Here's how the part is built. I have some questions about the finished solid (model axes, mm). Face numbers are marked on the shaded views. A direction names the side the tool comes from. Round coordinates to 2 decimals unless told otherwise and drop trailing zeros. Order: outer loops, then holes, each group sorted by start corner. A loop starts at its lowest first (then second) coordinate and runs counter-clockwise, first axis right, second up.
```python
from build123d import *

# Parameters (mm, degrees)
SKETCH1_R           = 7.5
SKETCH1_R_2         = 0.4
BOSS_EXTRUDE1_DEPTH = 2


with BuildPart() as part:
    # Sketch1 → Boss-Extrude1 (new body)
    with BuildSketch(Plane.XY):
        Circle(SKETCH1_R)
        with BuildLine():
            Line((-0.6, 6.723280449), (-0.6, 0.8))
            ThreePointArc((-0.6, 0.8), (-0.866025404, 0.5), (-0.992820323, 0.119615242))
            Line((-0.992820323, 0.119615242), (-6.122531666, -2.842024982))
            ThreePointArc((-6.122531666, -2.842024982), (-5.845671476, 3.375), (-0.6, 6.723280449))
        make_face(mode=Mode.SUBTRACT)
        with BuildLine():
            Line((-5.522531666, -3.881255467), (-0.392820323, -0.919615242))
            ThreePointArc((-0.392820323, -0.919615242), (0, -1), (0.392820323, -0.919615242))
            Line((0.392820323, -0.919615242), (5.522531666, -3.881255467))
            ThreePointArc((5.522531666, -3.881255467), (0, -6.75), (-5.522531666, -3.881255467))
        make_face(mode=Mode.SUBTRACT)
        with BuildLine():
            Line((6.122531666, -2.842024982), (0.992820323, 0.119615242))
            ThreePointArc((0.992820323, 0.119615242), (0.866025404, 0.5), (0.6, 0.8))
            Line((0.6, 0.8), (0.6, 6.723280449))
            ThreePointArc((0.6, 6.723280449), (5.845671476, 3.375), (6.122531666, -2.842024982))
        make_face(mode=Mode.SUBTRACT)
        Circle(SKETCH1_R_2, mode=Mode.SUBTRACT)
    extrude(amount=BOSS_EXTRUDE1_DEPTH)


solid = part.part
```
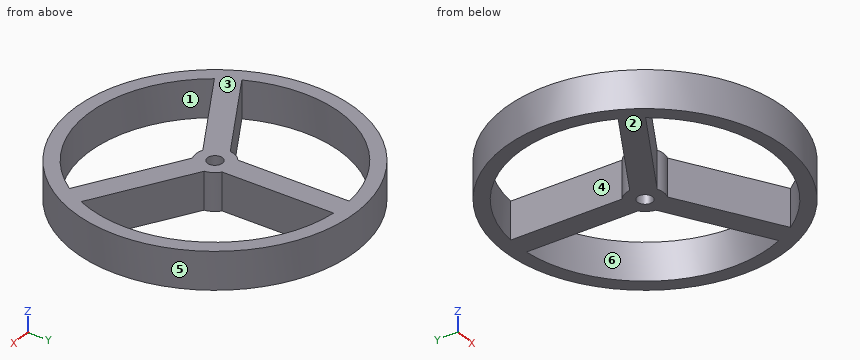
1. On a 3-axis mill with a long thin cutter (end or side, diameter ignored), from which of +Z, -Z, +X, -X, +Y, -Y can I reach the whole of each face in a straight line? I mean the marked faces 1 and 2. Say none if no direction works.
Evaluation:
face 1: +Z, -Z
face 2: -Z, +X, -X, +Y, -Y
2. I'm going to push flat-ended pins straight in: P1, Ø2, axis at x = -2, y = -3.5, coming from the -Z side; P2, Ø0.6, axis at y = 3, z = 0.5, coming from the +X side; P3, Ø1, axis at y = 4, z = 0.5, coming from the -X side. Where does each tip first touch, or does it pass through?
Evaluation:
P1: passes through
P2: stops at x = 7
P3: stops at x = -6.63
3. If we mould it in two halves opening along X, with no side actions, what happens to the marked faces 3, 4, 5 and 6? For each: released by +X, released by -X, zero draft, split by the parting line, or undercut.
Evaluation:
face 3: zero draft
face 4: undercut
face 5: split by the parting line
face 6: undercut
4. If we section it at B-B, the plane x = 0: Write out the boundary of the cut face in (y, z).
Evaluation:
outline: (-7.5, 0) - (-6.75, 0) - (-6.75, 2) - (-7.5, 2) - close; (-1, 0) - (-0.4, 0) - (-0.4, 2) - (-1, 2) - close; (0.4, 0) - (7.5, 0) - (7.5, 2) - (0.4, 2) - close
5. I need wall thicknesses on probe 1 along Y at (x, z) = (2, 0.9); probe 2 along X at (y, z) = (3.5, 0.4); probe 3 along Y at (x, z) = (-4, 0.95). Which ranges of each line are inside material? Lowest first, please.
Evaluation:
probe 1: y = -7.23 to -6.45, -1.85 to -0.46, 6.45 to 7.23
probe 2: x = -6.63 to -5.77, -0.6 to 0.6, 5.77 to 6.63
probe 3: y = -6.34 to -5.44, -3 to -1.62, 5.44 to 6.34
6. If we section it at A-A, the plane z = 0.4: Write out the boundary of the cut face in (x, y), and give its area (3 significant figures).
Evaluation:
outline: circle Ø15 at (0, 0); hole (-6.12, -2.84) - (-0.99, 0.12) arc R1 cw to (-0.6, 0.8) - (-0.6, 6.72) arc R6.75 ccw to start; hole (-5.52, -3.88) arc R6.75 ccw to (5.52, -3.88) - (0.39, -0.92) arc R1 cw to (-0.39, -0.92) - close; hole circle Ø0.8 at (0, 0); hole (0.6, 0.8) arc R1 cw to (0.99, 0.12) - (6.12, -2.84) arc R6.75 ccw to (0.6, 6.72) - close
area: 57.1 mm2
7. If we section it at C-C, the plane y = 6: Write out the boundary of the cut face in (x, z), and give its area (3 significant figures).
Evaluation:
outline: (-4.5, 0) - (-3.09, 0) - (-3.09, 2) - (-4.5, 2) - close; (-0.6, 0) - (0.6, 0) - (0.6, 2) - (-0.6, 2) - close; (3.09, 0) - (4.5, 0) - (4.5, 2) - (3.09, 2) - close
area: 8.03 mm2
